Check sheet for the modelled part. Datum: model origin and axes. Units: mm. A direction names the side the tool comes from. Coordinates: 2 decimals unless noted, no trailing zeros. Loops run counter-clockwise (first coordinate to the right, second up) from the corner with the lowest first, then second, coordinate; pieces in that order, holes last. Notation, with made-up numbers: M 35.5,83 L 68.5,83 A19 cw 68.5,115 Z; hole C 87.5,-32.75 d11. An arc over 180 degrees is marked long. Write each question's results on one line, items separated by ' | '. Start each with the question number.
from build123d import *

# Parameters (mm, degrees)
F0_R     = 5
F1_DEPTH = 5
F2_R     = 0.5
F3_DEPTH = 1.2
F2_R_2   = 2.5
F4_DEPTH = 1.2


with BuildPart() as f1:
    # F0 (on Top) → F1 (new body)
    with BuildSketch(Plane.XY):
        with Locations((-10.536088, 0)):
            Circle(F0_R)
    extrude(amount=F1_DEPTH)

    # F2 (on face) → F3 (join)
    with BuildSketch(Plane.XY.offset(5)):
        with Locations((-6.740328, 0)):
            Circle(F2_R)
        Polygon((-10.031058, -4.099747), (-10.031058, -3.516589), (-10.536088, -3.22501), (-11.041118, -3.516589), (-11.041118, -4.099747), (-10.536088, -4.391326), align=None)
    extrude(amount=F3_DEPTH)

    # F2 (on face) → F4 (cut)
    with BuildSketch(Plane.XY.offset(5)):
        with Locations((-10.536088, 0)):
            Circle(F2_R_2)
    extrude(amount=-F4_DEPTH, mode=Mode.SUBTRACT)


solid = f1.part
1) Section check D-D (z = 3.25). Enter the section's corners in (x, y), then the cut area to 3 significant figures.
2) Section check A-A (z = 5.75). Enter the section's corners in (x, y), then the cut area to 3 significant figures.
3) Set-up check for faces 4 (the flat face through (-11, 0, 0)), 5 (the cylindrical face through (-13.034, 0.11, 4.408)): record each of +Z, -Z, +X, -X, +Y, -Y from which the full face is reachable in a straight line by a thin tool's end or side.
4) Section check C-C (x = -12.25). Enter the section's corners in (y, z).
5) Gauge pin test, flat ends, axial feed: P1, Ø3, axis at y = -3.5, z = 4, coming from the +X side; P2, Ø4, axis at x = -10, y = 1, coming from the +Z side; P3, Ø0.6, axis at y = -4, z = 5.5, coming from the +X side; P4, Ø5, axis at x = -8, y = 2, coming from the -Z side. Record the tip position at first contact, or that the pin passes through.
6) Release check for a two-part mould opening along Y. For faces 1 (the cylindrical face through (-7.24, 0.02, 5.59)), 2 (the flat face through (-10.5, -3.8, 6.2)), 3 (the flat face through (-11, 0, 3.8)) record: +Y half, -Y half, draft (parallel to the pull), parting line (faces both ways), or undercut.
7) Thickness scan on probe 1 along Y at (x, z) = (-10.5, 4); probe 2 along Z at (x, y) = (-13.75, -2.5); probe 3 along Y at (x, z) = (-12.25, 4.25). Record the ranges inside material, lowest first.
8) Section check B-B (y = 0). Enter the section's corners in (x, z).
Return value:
1) outline: C -10.54,0 d10 | area: 78.5 mm2
2) outline: M -11.04,-4.1 L -10.54,-4.39 L -10.03,-4.1 L -10.03,-3.52 L -10.54,-3.23 L -11.04,-3.52 Z; C -6.74,0 d1 | area: 1.67 mm2
3) face 4: -Z, +X, -X, +Y, -Y | face 5: +Z
4) outline: M -4.7,0 L 4.7,0 L 4.7,5 L 1.82,5 L 1.82,3.8 L -1.82,3.8 L -1.82,5 L -4.7,5 Z
5) P1: stops at x = -5.95 | P2: stops at z = 5 | P3: stops at x = -10.03 | P4: stops at z = 0
6) face 1: parting line | face 2: draft | face 3: undercut
7) probe 1: y = -5 to -2.5, 2.5 to 5 | probe 2: z = 0 to 5 | probe 3: y = -4.7 to -1.82, 1.82 to 4.7
8) outline: M -15.54,0 L -5.54,0 L -5.54,5 L -6.24,5 L -6.24,6.2 L -7.24,6.2 L -7.24,5 L -8.04,5 L -8.04,3.8 L -13.04,3.8 L -13.04,5 L -15.54,5 Z
